```python
from build123d import *

# Parameters (mm, degrees)
SKETCH016_W      = 6.6
SKETCH016_H      = 6.8
PAD007_DEPTH     = 8.5
CHAMFER004_SIZE2 = 1.4
CHAMFER004_SIZE  = 3.7
CHAMFER005_SIZE2 = 3.7
CHAMFER005_SIZE  = 1.4


with BuildPart() as part:
    # Sketch016 → Pad007 (new body)
    with BuildSketch(Plane.XY):
        with Locations((50.1, 20.6)):
            Rectangle(SKETCH016_W, SKETCH016_H)
    extrude(amount=PAD007_DEPTH)

    # Chamfer004
    chamfer004_edges = [part.edges().sort_by_distance(p)[0] for p in [
        (53.4, 20.6, 8.5),
    ]]
    chamfer004_side = part.faces().sort_by_distance((53.4, 20.6, 4.25))[0]
    chamfer(chamfer004_edges, length=CHAMFER004_SIZE, length2=CHAMFER004_SIZE2, reference=chamfer004_side)

    # Chamfer005
    chamfer005_edges = [part.edges().sort_by_distance(p)[0] for p in [
        (46.8, 20.6, 8.5),
    ]]
    chamfer005_side = part.faces().sort_by_distance((49.4, 20.6, 8.5))[0]
    chamfer(chamfer005_edges, length=CHAMFER005_SIZE, length2=CHAMFER005_SIZE2, reference=chamfer005_side)


with BuildPart() as part_1:
    # Body020 placement: moved
    add(part.part.moved(Location((-26.7, 0, 0))))


solid = part_1.part
```
For this review, take the finished solid that the model builds, in its own axes (mm). Round coordinates to 2 decimals unless told otherwise and drop trailing zeros. Write each loop counter-clockwise with the first axis right and the second up, starting at its lowest first coordinate (ties: lowest second). Pieces come first, ordered by that corner, then holes. Notation, with made-up numbers: (78.5, 31.5) - (84.5, 31.5) arc R12 ccw to (84.5, 49.5) - close; hole circle Ø1 at (51.25, -20). An arc over 180 degrees is marked (long way). Answer as CSV lines item,"result". Start each with the question number.
(1) Add section C-C, the plane z = 5.75. State the section outline as (x, y) points.
(2) For line 1 (X direction, y = 22.25, z = 5.25); line 2 (X direction, y = 18, z = 5), list the stretches that pass through material, from the lowest coordinate up.
(3) Add section A-A, the plane y = 18.5. State the section outline as (x, z) points, plus the area to 3 significant figures.
(4) Add section B-B, the plane x = 26. State the section outline as (y, z) points.
From the geometry:
1,outline,"(20.46, 17.2) - (26.34, 17.2) - (26.34, 24) - (20.46, 24) - close"
2,line 1,"x = 20.27 to 26.53"
2,line 2,"x = 20.18 to 26.62"
3,outline,"(20.1, 0) - (26.7, 0) - (26.7, 4.8) - (25.3, 8.5) - (21.5, 8.5) - (20.1, 4.8) - close"
3,area,"50.9 mm²"
4,outline,"(17.2, 0) - (24, 0) - (24, 6.65) - (17.2, 6.65) - close"
